Geometry check sheet. Reference: drawing and pictorial views, mm from the part's lowest x, y, z. A direction names the side the tool comes from. Coordinates: 2 decimals unless noted, no trailing zeros. Write each loop counter-clockwise with the first axis right and the second up, starting at its lowest first coordinate (ties: lowest second). Pieces come first, ordered by that corner, then holes. Notation, with made-up numbers: (6, 6) -> (17, 6) arc R35 cw to (17, 39) -> close; hole circle Ø10 at (-34.5, 21). An arc over 180 degrees is marked (long way). Put each result on its own line as item: value.
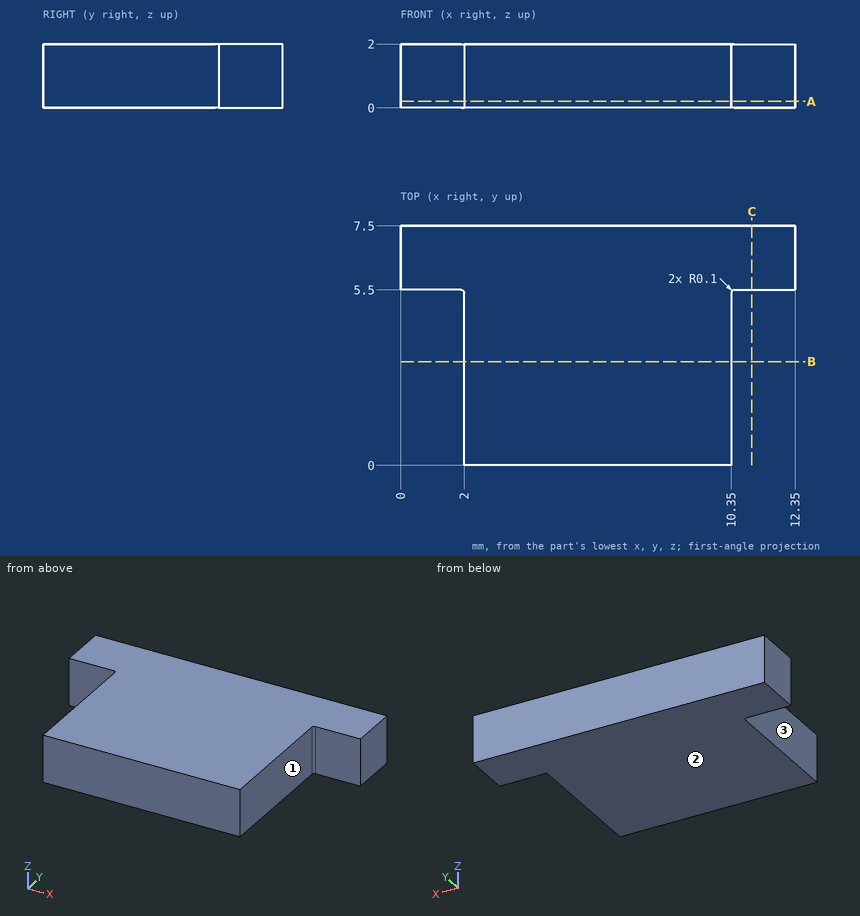
Q1. Cross-section at C-C (x = 11). Record the cut outline in (y, z), plus the area to 3 significant figures.
Recorded:
outline: (5.5, 0) -> (7.5, 0) -> (7.5, 2) -> (5.5, 2) -> close
area: 4.00 mm2
Q2. Cross-section at B-B (y = 3.25). Record the cut outline in (x, z).
Recorded:
outline: (2, 0) -> (10.35, 0) -> (10.35, 2) -> (2, 2) -> close
Q3. Depth check by flat-ended pin: P1, Ø0.6, axis at x = 1, z = 1, coming from the -Y side. Enter the tip coordinate at first touch or a pass-through.
Recorded:
P1: stops at y = 5.5
Q4. Cross-section at A-A (z = 0.2). Record the cut outline in (x, y).
Recorded:
outline: (0, 5.5) -> (1.9, 5.5) arc R0.1 cw to (2, 5.4) -> (2, 0) -> (10.35, 0) -> (10.35, 5.4) arc R0.1 cw to (10.45, 5.5) -> (12.35, 5.5) -> (12.35, 7.5) -> (0, 7.5) -> close
Q5. Tool access check on the marked faces 1, 2 and 3. Record the directions out of +Z, -Z, +X, -X, +Y, -Y that give a thin tool (end or side, any length) a straight path to the whole face; none if there is none.
Recorded:
face 1: +Z, -Z, +X, -Y
face 2: -Z, +X, -X, +Y, -Y
face 3: +Z, -Z, -X, -Y
Q6. Material ranges on line 1 along Y through (x, z) = (11, 0.3); line 2 along X through (y, z) = (2.25, 0.8), recorded low to high.
Recorded:
line 1: y = 5.5 to 7.5
line 2: x = 2 to 10.35
